The listing builds one solid part. Answer for the finished solid, in the listing's coordinates (mm). Round coordinates to 2 decimals unless told otherwise and drop trailing zeros. Order: outer loops, then holes, each group sorted by start corner. A loop starts at its lowest first (then second) coordinate and runs counter-clockwise, first axis right, second up. Notation, with made-up numbers: (15, 22) - (27, 22) arc R29 cw to (27, 46) - close; hole circle Ø9 at (37.5, -11.75). An arc over 180 degrees is marked (long way). Use CSV: the item, a comma, the result in double quotes. Start each with the question number.
Item 1: Determine the mould class of faces 1 (the conical face through (86.431, 8.214, 4.896)), 2 (the flat face through (44.245, -7.785, -5.061)), 3 (the conical face through (86.431, 0.133, -9.562)) for opening direction Z: +Z half, -Z half, draft (parallel to the pull), parting line (faces both ways), or undercut.
Item 2: Find section A-A, the plane x = 17. Give the vertices of the cut face in (y, z).
Item 3: Flat-ended cylindrical pins translate along their axes: P1, Ø1, axis at x = 80.5, y = 2.5, coming from the +Z side; P2, Ø3, axis at x = 50.5, z = -5, coming from the +Y side; P3, Ø2, axis at y = -4.5, z = 7.5, coming from the +X side. Find the tip coordinate at first contact, or state that the pin passes through.
Item 4: Straight lines are drawn through the part: line 1 along Y through (x, z) = (51.5, -3.75); line 2 along Z through (x, y) = (82.5, -0.5); line 3 along X through (y, z) = (6.75, -3.25). For each, find the intervals that lie inside material, in ascending order. Write a range as [from, to].
Autodesk Inventor part; units mm, degrees
ref_plane "YZ Plane" through (0, 0, 0) normal (1, 0, 0) x (0, 1, 0)
ref_plane "XZ Plane" through (0, 0, 0) normal (0, 1, 0) x (-1, 0, 0)
ref_plane "XY Plane" through (0, 0, 0) normal (0, 0, 1) x (1, 0, 0)
sketch "Sketch1" plane through (0, 0, 0) normal (0, 0, 1) x (1, 0, 0)
  line L0 (87.5, 9.2765) -> (84.8, 10)
  line L1 (84.8, 10) -> (2.5, 10)
  line L2 (0, 0) -> (90, 0)
  arc A0 (90, 0) -> (87.5, 9.2765) centre (71.5392, 0) ccw
  arc A1 (2.5, 10) -> (0, 0) centre (21.25, 0) ccw
  dimension "d0" = 90
  dimension "d1" = 20
  dimension "d2" = 5.2
  dimension "d3" = 15
  dimension "d4" = 2.5
  dimension "d5" = 2.5
revolve "Body" add sketch "Sketch1" angle 360 about axis through (0, 0, 0) along (1, 0, 0)
sketch "Sketch2" plane through (0, 0, 0) normal (1, 0, 0) x (0, 1, 0)
  circle A0 centre (0, 0) radius 10
  line L0 (0, 10) -> (-1, 10)
  line L1 (0, 10) -> (1, 10)
  line L2 (-1, 10) -> (0, 8.5719)
  line L3 (0, 8.5719) -> (1, 10)
  line L4 (0, -14) -> (0, 14)
  dimension "d6" = 35
  dimension "d7" = 35
  dimension "d8" = 1
extrude "Groove" cut sketch "Sketch2" along normal through all contours L3 L4 A0 | A0 L1 L3 | L4 L2 A0 | A0 L2 L0 picked at (0.5375, 9.5014) picked at (-0.5375, 9.5014)
pattern_circular "Grooves" count 3 over 360 about axis through (-10, 0, 0) along (1, 0, 0) of "Groove"
equation "\"d0\" = NLG"
equation "\"d1\" = NND"
equation "\"d2\" = PHH"
equation "\"d3\" = FAWI"
equation "\"d4\" = KAH"
equation "\"d5\" = KAH"
equation "\"d8\" = 0.05 * NND"
equation "\"NND\" = 20"
equation "\"NLG\" = 90"
equation "\"PHH\" = 5.2"
equation "\"FAWI\" = 15deg"
equation "\"KAH\" = 2.5"
equation "\"d13\" = -KAH"
equation "\"d28\" = KAH"
equation "\"NND1\" = 20.5"
equation "\"KAH1\" = 1.82"
equation "\"NLG1\" = 88.18"
properties part number "CNS 9215 - 20 x 90" material "Steel, Mild"
Worked out:
1,face 1,"parting line"
1,face 2,"undercut"
1,face 3,"-Z half"
2,outline,"(-9.1, -4.14) - (-7.42, -4.29) - (-8.14, -5.81) arc R10 ccw to (8.14, -5.81) - (7.42, -4.29) - (9.1, -4.14) arc R10 ccw to (0.97, 9.95) - (0, 8.57) - (-0.97, 9.95) arc R10 ccw to start"
3,P1,"stops at z = 9.8"
3,P2,"stops at y = 9.37"
3,P3,"stops at x = 88.3"
4,line 1,"y = [-9.27, 9.27]"
4,line 2,"z = [-9.99, 9.29]"
4,line 3,"x = [1.36, 88.41]"
